Geometry: final body of the model. Coordinates: model frame, mm. Coordinates: 2 decimals unless noted, no trailing zeros. Put each result on its own line as item: value. Start each with the question number.
1) Material intervals for line 1 along X through (y, z) = (-0.1, 0); line 2 along X through (y, z) = (2.35, -18.5); line 3 along X through (y, z) = (2.2, -16.5), sorted ascending. Write a range as from..to.
2) Draft query along X for faces 1 (the cylindrical face through (6.665, 1.479, 20.966)), 2 (the cylindrical face through (21.047, 1.479, -12.756)). Return one class per face: +X half, -X half, draft (parallel to the pull), parting line (faces both ways), or undercut.
3) Section A-A on y = 0.65. Count the separate pieces of the cut face and the enclosed holes in it, and give its area (3 significant figures).
4) Contact query for a flat-ended pin moving along its axis: pin 1 Ø1.9 at (x, z) = (0, 0) entering from +Y. Output: stop coordinate, or through.
```python
from build123d import *

# Parameters (mm, degrees)
EXTRUDE_1_DEPTH     = 3
EXTRUDE_1_2_DEPTH   = 3
EXTRUDE_1_3_DEPTH   = 3
EXTRUDE_1_4_DEPTH   = 3
SKETCH_1_R          = 35
EXTRUDE_1_5_DEPTH   = 3
SKETCH_3_R          = 35
EXTRUDE_2_DEPTH     = 1
SKETCH_4_R          = 1.55
CUT_EXTRUDE_1_DEPTH = 5


with BuildPart() as part:
    # Sketch 1 → Extrude 1 (new body)
    with BuildSketch(Plane(origin=(0, 0, 0), x_dir=(1, 0, 0), z_dir=(0, 1, 0))):
        with BuildLine():
            ThreePointArc((-8.987940463, 4.383711468), (-8.595708593, 6.301111944), (-9.178240759, 8.169514123))
            ThreePointArc((-9.178240759, 8.169514123), (-9.312956952, 8.786525533), (-9.030558816, 9.351417404))
            ThreePointArc((-9.030558816, 9.351417404), (-7.64120828, 10.517220927), (-6.103130316, 11.478318707))
            ThreePointArc((-6.103130316, 11.478318707), (-5.224804474, 11.603054959), (-4.470435457, 11.136211511))
            ThreePointArc((-4.470435457, 11.136211511), (-3.095389379, 10.109363067), (-1.39173101, 9.902680687))
            ThreePointArc((-1.39173101, 9.902680687), (3.090169944, 9.510565163), (6.946583705, 7.193398003))
            ThreePointArc((6.946583705, 7.193398003), (8.648933609, 6.227853996), (10.605902015, 6.204506982))
            ThreePointArc((10.605902015, 6.204506982), (11.23434433, 6.141962683), (11.684322602, 5.698824908))
            ThreePointArc((11.684322602, 5.698824908), (12.363734712, 4.017220927), (12.802500789, 2.25742631))
            ThreePointArc((12.802500789, 2.25742631), (12.649714402, 1.383543172), (11.972607053, 0.810358162))
            ThreePointArc((11.972607053, 0.810358162), (10.571103543, -0.180074751), (9.84807753, -1.736481777))
            ThreePointArc((9.84807753, -1.736481777), (-3.090169944, -9.510565163), (-8.987940463, 4.383711468))
        make_face()
    extrude(amount=EXTRUDE_1_DEPTH)



with BuildPart() as body_2:
    # Sketch 1 → Extrude 1 2 (new body)
    with BuildSketch(Plane(origin=(0, 0, 0), x_dir=(1, 0, 0), z_dir=(0, 1, 0))):
        with BuildLine():
            ThreePointArc((-11.114533927, -11.509436805), (-12.492455263, -10.599830784), (-14.105693288, -10.248386061))
            ThreePointArc((-14.105693288, -10.248386061), (-15.858793025, -9.702695478), (-17.07708688, -8.329051789))
            ThreePointArc((-17.07708688, -8.329051789), (-19, 0), (-17.07708688, 8.329051789))
            ThreePointArc((-17.07708688, 8.329051789), (-15.858793025, 9.702695478), (-14.105693288, 10.248386061))
            ThreePointArc((-14.105693288, 10.248386061), (-12.492455263, 10.599830784), (-11.114533927, 11.509436805))
            ThreePointArc((-11.114533927, 11.509436805), (16, 0), (-11.114533927, -11.509436805))
        make_face()
        with BuildLine():
            ThreePointArc((-10.785528556, 5.260453761), (-3.708203932, -11.412678196), (11.817693036, -2.083778132))
            ThreePointArc((11.817693036, -2.083778132), (12.10690446, -1.461213129), (12.667507838, -1.065038569))
            ThreePointArc((12.667507838, -1.065038569), (14.384650397, 0.388557195), (14.772116295, 2.604722665))
            ThreePointArc((14.772116295, 2.604722665), (14.265847744, 4.635254916), (13.481910694, 6.575567202))
            ThreePointArc((13.481910694, 6.575567202), (12.083449441, 7.952769275), (10.130350184, 8.147147056))
            ThreePointArc((10.130350184, 8.147147056), (9.17069564, 8.158595921), (8.335900446, 8.632077604))
            ThreePointArc((8.335900446, 8.632077604), (3.708203932, 11.412678196), (-1.670077212, 11.883216825))
            ThreePointArc((-1.670077212, 11.883216825), (-2.351542959, 11.965890068), (-2.901563328, 12.376630892))
            ThreePointArc((-2.901563328, 12.376630892), (-4.814641283, 13.560544718), (-7.042073442, 13.244213893))
            ThreePointArc((-7.042073442, 13.244213893), (-8.816778784, 12.135254916), (-10.419875557, 10.790097005))
            ThreePointArc((-10.419875557, 10.790097005), (-11.297524269, 9.034502472), (-10.878847662, 7.116928659))
            ThreePointArc((-10.878847662, 7.116928659), (-10.593186617, 6.200705058), (-10.785528556, 5.260453761))
        make_face(mode=Mode.SUBTRACT)
    extrude(amount=EXTRUDE_1_2_DEPTH)


with BuildPart() as body_3:
    # Sketch 1 → Extrude 1 3 (new body)
    with BuildSketch(Plane(origin=(0, 0, 0), x_dir=(1, 0, 0), z_dir=(0, 1, 0))):
        with BuildLine():
            ThreePointArc((18.937750033, -13.8084093), (21.021041042, -12.777130739), (22.469851157, -10.95927867))
            ThreePointArc((22.469851157, -10.95927867), (25, 0), (22.469851157, 10.95927867))
            ThreePointArc((22.469851157, 10.95927867), (21.021041042, 12.777130739), (18.937750033, 13.8084093))
            ThreePointArc((18.937750033, 13.8084093), (16.976365134, 14.574561246), (15.28248415, 15.825475607))
            ThreePointArc((15.28248415, 15.825475607), (-12.93127555, 17.798373876), (-19.773469019, -9.644165229))
            ThreePointArc((-19.773469019, -9.644165229), (-19.107216775, -11.641695573), (-18.98466424, -13.743837434))
            ThreePointArc((-18.98466424, -13.743837434), (-18.647632371, -16.043847525), (-17.366459261, -17.983495008))
            ThreePointArc((-17.366459261, -17.983495008), (-14.694631307, -20.225424859), (-11.73678907, -22.073689821))
            ThreePointArc((-11.73678907, -22.073689821), (-9.496170427, -22.69277382), (-7.204582268, -22.302567971))
            ThreePointArc((-7.204582268, -22.302567971), (-5.167455737, -21.769524797), (-3.061808221, -21.785897512))
            ThreePointArc((-3.061808221, -21.785897512), (6.798373876, -20.923243358), (15.28248415, -15.825475607))
            ThreePointArc((15.28248415, -15.825475607), (16.976365134, -14.574561246), (18.937750033, -13.8084093))
        make_face()
        with BuildLine():
            ThreePointArc((-12.503850668, -12.948116406), (-13.269414492, -12.44274542), (-14.165718687, -12.247485096))
            ThreePointArc((-14.165718687, -12.247485096), (-16.943967267, -11.382694545), (-18.874674972, -9.205794083))
            ThreePointArc((-18.874674972, -9.205794083), (-21, 0), (-18.874674972, 9.205794083))
            ThreePointArc((-18.874674972, 9.205794083), (-16.943967267, 11.382694545), (-14.165718687, 12.247485096))
            ThreePointArc((-14.165718687, 12.247485096), (-13.269414492, 12.44274542), (-12.503850668, 12.948116406))
            ThreePointArc((-12.503850668, 12.948116406), (18, 0), (-12.503850668, -12.948116406))
        make_face(mode=Mode.SUBTRACT)
    extrude(amount=EXTRUDE_1_3_DEPTH)


with BuildPart() as body_4:
    # Sketch 1 → Extrude 1 4 (new body)
    with BuildSketch(Plane(origin=(0, 0, 0), x_dir=(1, 0, 0), z_dir=(0, 1, 0))):
        with BuildLine():
            ThreePointArc((-4.31436613, 30.698310131), (18.221342821, 25.079526826), (30.529040343, 5.383093508))
            ThreePointArc((30.529040343, 5.383093508), (30.48111684, 2.285468824), (29.287623908, -0.573403325))
            ThreePointArc((29.287623908, -0.573403325), (28.210037241, -2.62947128), (27.574617084, -4.862148975))
            ThreePointArc((27.574617084, -4.862148975), (16.457987064, -22.652475842), (-3.896846827, -27.727505925))
            ThreePointArc((-3.896846827, -27.727505925), (-5.993969283, -27.657741779), (-8.058542774, -28.03234281))
            ThreePointArc((-8.058542774, -28.03234281), (-11.37088699, -28.338686756), (-14.553618446, -27.371375379))
            ThreePointArc((-14.553618446, -27.371375379), (-18.221342821, -25.079526826), (-21.534409484, -22.29953381))
            ThreePointArc((-21.534409484, -22.29953381), (-23.316376662, -19.765334071), (-24.031223485, -16.750940373))
            ThreePointArc((-24.031223485, -16.750940373), (-24.36796398, -14.454156905), (-25.166233296, -12.27439211))
            ThreePointArc((-25.166233296, -12.27439211), (-26.629582456, 8.652475843), (-13.145203758, 24.7225326))
            ThreePointArc((-13.145203758, 24.7225326), (-11.218156715, 26.016788431), (-9.595712481, 27.676994193))
            ThreePointArc((-9.595712481, 27.676994193), (-7.245573093, 29.695513501), (-4.31436613, 30.698310131))
        make_face()
        with BuildLine():
            ThreePointArc((24.26743925, -11.836020963), (27, 0), (24.26743925, 11.836020963))
            ThreePointArc((24.26743925, 11.836020963), (22.276722717, 14.333814244), (19.414206911, 15.750827598))
            ThreePointArc((19.414206911, 15.750827598), (17.942654929, 16.325642065), (16.671800891, 17.264155208))
            ThreePointArc((16.671800891, 17.264155208), (-14.106846055, 19.416407865), (-21.571057111, -10.520907523))
            ThreePointArc((-21.571057111, -10.520907523), (-21.071193566, -12.019578048), (-20.979247092, -13.596734588))
            ThreePointArc((-20.979247092, -13.596734588), (-20.516153338, -16.757030106), (-18.755776002, -19.422174609))
            ThreePointArc((-18.755776002, -19.422174609), (-15.870201812, -21.843458848), (-12.675732195, -23.839585007))
            ThreePointArc((-12.675732195, -23.839585007), (-9.597042635, -24.6902284), (-6.448319149, -24.15407171))
            ThreePointArc((-6.448319149, -24.15407171), (-4.919941122, -23.754149829), (-3.340154423, -23.76643365))
            ThreePointArc((-3.340154423, -23.76643365), (7.416407865, -22.825356391), (16.671800891, -17.264155208))
            ThreePointArc((16.671800891, -17.264155208), (17.942654929, -16.325642065), (19.414206911, -15.750827598))
            ThreePointArc((19.414206911, -15.750827598), (22.276722717, -14.333814244), (24.26743925, -11.836020963))
        make_face(mode=Mode.SUBTRACT)
    extrude(amount=EXTRUDE_1_4_DEPTH)


with BuildPart() as body_5:
    # Sketch 1 → Extrude 1 5 (new body)
    with BuildSketch(Plane(origin=(0, 0, 0), x_dir=(1, 0, 0), z_dir=(0, 1, 0))):
        Circle(SKETCH_1_R)
        with BuildLine():
            ThreePointArc((-4.592712332, 32.678846268), (-8.238694275, 31.431517625), (-11.161915282, 28.920782272))
            ThreePointArc((-11.161915282, 28.920782272), (-12.497644107, 27.553965069), (-14.084146884, 26.488427786))
            ThreePointArc((-14.084146884, 26.488427786), (-28.531695489, 9.270509831), (-26.963821389, -13.151134404))
            ThreePointArc((-26.963821389, -13.151134404), (-26.306620782, -14.945695108), (-26.029388457, -16.836595159))
            ThreePointArc((-26.029388457, -16.836595159), (-25.140226197, -20.586048925), (-22.923726225, -23.738213411))
            ThreePointArc((-22.923726225, -23.738213411), (-19.396913326, -26.697560814), (-15.492561572, -29.137270564))
            ThreePointArc((-15.492561572, -29.137270564), (-11.698213434, -30.314961384), (-7.736329089, -30.019147427))
            ThreePointArc((-7.736329089, -30.019147427), (-5.969810062, -29.709434307), (-4.176359771, -29.716343862))
            ThreePointArc((-4.176359771, -29.716343862), (17.759481282, -24.44665794), (29.54423259, -5.20944533))
            ThreePointArc((29.54423259, -5.20944533), (30.067362447, -3.371322398), (30.954519948, -1.678599051))
            ThreePointArc((30.954519948, -1.678599051), (32.439046197, 1.87740923), (32.498655849, 5.730389863))
            ThreePointArc((32.498655849, 5.730389863), (19.396913326, 26.697560814), (-4.592712332, 32.678846268))
        make_face(mode=Mode.SUBTRACT)
    extrude(amount=EXTRUDE_1_5_DEPTH)


with BuildPart() as part_1:
    add(part.part)

    add(body_2.part)  # Extrude 2 merges body 2

    add(body_3.part)  # Extrude 2 merges body 3

    add(body_4.part)  # Extrude 2 merges body 4

    add(body_5.part)  # Extrude 2 merges body 5
    # Sketch 3 → Extrude 2 (add)
    with BuildSketch(Plane.XZ):
        Circle(SKETCH_3_R)
    extrude(amount=EXTRUDE_2_DEPTH)

    # Sketch 4 → Cut-Extrude 1 (cut, through all)
    with BuildSketch(Plane(origin=(0, 3, 0), x_dir=(1, 0, 0), z_dir=(0, 1, 0))):
        Circle(SKETCH_4_R)
    extrude(amount=-CUT_EXTRUDE_1_DEPTH, mode=Mode.SUBTRACT)


solid = part_1.part
```
Answer block:
1. line 1: x = -35..-1.55, 1.55..35
1. line 2: x = -29.71..-23.62, -21.02..-15.29, -11.91..11.91, 15.29..24.87, 27.33..29.71
1. line 3: x = -30.87..-25.05, -22.62..-17.43, -14.55..-7.19, 7.19..14.55, 17.65..26.24, 28.58..30.87
2. face 1: undercut
2. face 2: undercut
3. separate pieces: 5
3. enclosed holes: 5
3. area: 2,760 mm²
4. pin 1: passes through
